Read the model definition and answer for the solid it produces. Units are mm, in the model's axes. Face numbers are marked on the shaded views. A direction names the side the tool comes from. Give positions to 0.01 mm unless a question says otherwise; leave off trailing zeros. Loops run counter-clockwise (first coordinate to the right, second up) from the corner with the lowest first, then second, coordinate; pieces in that order, holes last.
(1) Straight lines are drawn through the part: probe 1 along Z at (x, y) = (25.5, 17); probe 2 along Y at (x, z) = (16, -4); probe 3 along Z at (x, y) = (-20, 5.75). For each, find the intervals that lie inside material, in ascending order.
(2) Find section D-D, the plane z = 24. Write down the section's boundary in (x, y).
(3) Which of the six approach directions +Z, -Z, +X, -X, +Y, -Y give full straight-line access (tool end or side, diameter ignored) to the marked faces 1 and 2?
(4) Each of these flat-tipped pins is pushed along its axis until it touches: P1, Ø2.5, axis at x = 29.8, y = 13, coming from the +Z side; P2, Ø5, axis at x = 27.5, y = 13, coming from the +Z side; P3, Ø9, axis at x = 19.8, z = 13.34, coming from the -Y side; P4, Ø13, axis at x = -20.2, z = 13.34, coming from the +Y side. Where does it stop, or does it pass through?
(5) Find section B-B, the plane x = 30. Write down the section's boundary in (y, z), then the cut area to 3 significant figures.
(6) Find section A-A, the plane y = 13. Write down the section's boundary in (x, z), then the cut area to 3 significant figures.
(7) Find section C-C, the plane y = 1.5. Write down the section's boundary in (x, z).
```python
from build123d import *

# Parameters (mm, degrees)
SKETCH1_W                 = 80
SKETCH1_H                 = 40
BOSS_EXTRUDE1_DEPTH       = 8
SKETCH2_R                 = 4
CUT_EXTRUDE1_DEPTH        = 4
SKETCH3_W                 = 20
SKETCH3_H                 = 5
BOSS_EXTRUDE2_DEPTH       = 10
SKETCH5_R                 = 5.75
CUT_EXTRUDE3_DEPTH        = 4
F_8_CLEARANCE_HOLE1_D     = 4.4958
F_8_CLEARANCE_HOLE1_DEPTH = 5
F_8_CLEARANCE_HOLE1_TIP   = 1.350674586


with BuildPart() as part:
    # Sketch1 → Boss-Extrude1 (new body)
    with BuildSketch(Plane(origin=(0, 0, 0), x_dir=(1, 0, 0), z_dir=(0, 1, 0))):
        with Locations((-0.202602356, -13.338458494)):
            Rectangle(SKETCH1_W, SKETCH1_H)
    extrude(amount=BOSS_EXTRUDE1_DEPTH)

    # Sketch2 → Cut-Extrude1 (cut)
    with BuildSketch(Plane(origin=(0, 8, 0), x_dir=(1, 0, 0), z_dir=(0, 1, 0))):
        with Locations((19.797397644, -13.338458494)):
            Circle(SKETCH2_R)
        with Locations((-20.202602356, -13.338458494)):
            Circle(SKETCH2_R)
    extrude(amount=-CUT_EXTRUDE1_DEPTH, mode=Mode.SUBTRACT)

    # Sketch3 → Boss-Extrude2 (add)
    with BuildSketch(Plane(origin=(0, 8, 0), x_dir=(1, 0, 0), z_dir=(0, 1, 0))):
        with Locations((29.797397644, 4.161541506)):
            Rectangle(SKETCH3_W, SKETCH3_H)
        with Locations((-30.202602356, 4.161541506)):
            Rectangle(SKETCH3_W, SKETCH3_H)
    extrude(amount=BOSS_EXTRUDE2_DEPTH)

    # Sketch5 → Cut-Extrude3 (cut)
    with BuildSketch(Plane(origin=(0, 0, 0), x_dir=(-1, 0, 0), z_dir=(0, -1, 0))):
        with Locations((20.202602356, -13.338458494)):
            Circle(SKETCH5_R)
        with Locations((-19.797397644, -13.338458494)):
            Circle(SKETCH5_R)
    extrude(amount=-CUT_EXTRUDE3_DEPTH, mode=Mode.SUBTRACT)

    # #8 Clearance Hole1
    with Locations(Plane(origin=(29.797397644, 13, -6.661541506), x_dir=(-1, 0, 0), z_dir=(0, 0, -1))):
        with Locations((0, 0), (60, 0)):
            Hole(F_8_CLEARANCE_HOLE1_D / 2, depth=F_8_CLEARANCE_HOLE1_DEPTH)
            with Locations((0, 0, -(F_8_CLEARANCE_HOLE1_DEPTH + F_8_CLEARANCE_HOLE1_TIP / 2))):  # 118° drill point
                Cone(0, F_8_CLEARANCE_HOLE1_D / 2, F_8_CLEARANCE_HOLE1_TIP, mode=Mode.SUBTRACT)


solid = part.part
```
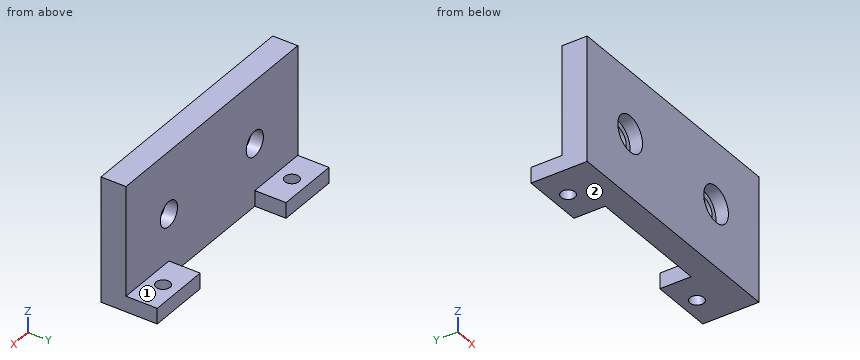
Entries:
1. probe 1: z = -6.66 to -1.66
1. probe 2: y = 0 to 8
1. probe 3: z = -6.66 to 9.34, 17.33 to 33.34
2. outline: (-40.2, 0) - (39.8, 0) - (39.8, 8) - (-40.2, 8) - close
3. face 1: +Z, +X, -X, +Y
3. face 2: -Z, +X, -X, +Y, -Y
4. P1: passes through
4. P2: stops at z = -1.66
4. P3: stops at y = 4
4. P4: stops at y = 8
5. outline: (0, -6.66) - (10.76, -6.66) - (10.76, -1.66) - (8, -1.66) - (8, 33.34) - (0, 33.34) - close; (15.24, -6.66) - (18, -6.66) - (18, -1.66) - (15.24, -1.66) - close
5. area: 348 mm2
6. outline: (-40.2, -6.66) - (-32.45, -6.66) - (-32.45, -1.66) - (-40.2, -1.66) - close; (-27.95, -6.66) - (-20.2, -6.66) - (-20.2, -1.66) - (-27.95, -1.66) - close; (19.8, -6.66) - (27.55, -6.66) - (27.55, -1.66) - (19.8, -1.66) - close; (32.05, -6.66) - (39.8, -6.66) - (39.8, -1.66) - (32.05, -1.66) - close
6. area: 155 mm2
7. outline: (-40.2, -6.66) - (39.8, -6.66) - (39.8, 33.34) - (-40.2, 33.34) - close; hole circle Ø11.5 at (-20.2, 13.34); hole circle Ø11.5 at (19.8, 13.34)
